For this review, use the dimensioned drawing (mm, ordinates from the lowest corner) and the shaded views. Round coordinates to 2 decimals unless told otherwise and drop trailing zeros. Write each loop counter-clockwise with the first axis right and the second up, starting at its lowest first coordinate (ties: lowest second). Pieces come first, ordered by that corner, then holes.
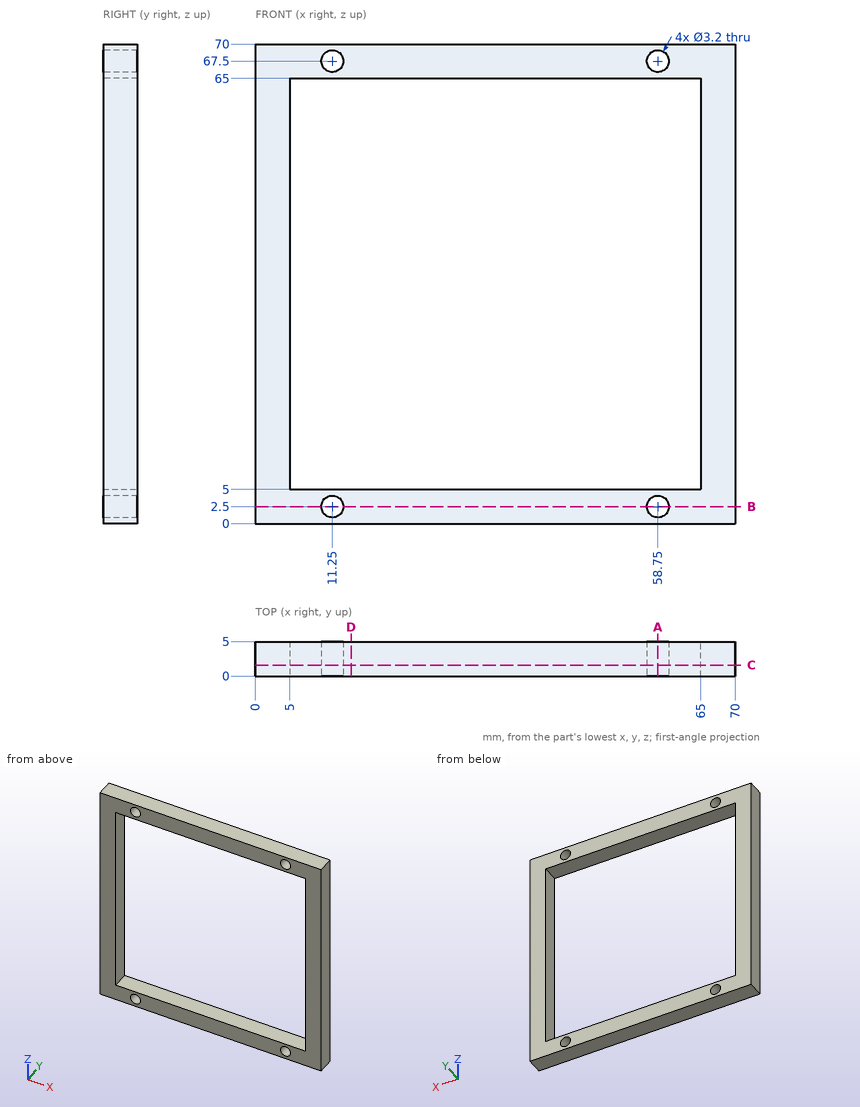
(1) We need section C-C, the plane y = 1.6. Give the boundary of the cut face in (x, z), and give its area (3 significant figures).
Geometry check:
outline: (0, 0) - (70, 0) - (70, 70) - (0, 70) - close; hole (5, 5) - (65, 5) - (65, 65) - (5, 65) - close; hole circle Ø3.2 at (11.25, 2.5); hole circle Ø3.2 at (11.25, 67.5); hole circle Ø3.2 at (58.75, 2.5); hole circle Ø3.2 at (58.75, 67.5)
area: 1,270 mm2
(2) For line 1 along Z through (x, y) = (58.75, 3.95); line 2 along X through (y, z) = (3.75, 51), list the stretches that pass through material, from the lowest coordinate up.
Geometry check:
line 1: z = 0 to 0.9, 4.1 to 5, 65 to 65.9, 69.1 to 70
line 2: x = 0 to 5, 65 to 70
(3) For pin 1 Ø1.9 at (x, z) = (58.75, 67.5) entering from -Y; pin 2 Ø1 at (y, z) = (3, 57) entering from -X, all flat-tipped, find the tip position at first contact; note any pin that passes through.
Geometry check:
pin 1: passes through
pin 2: stops at x = 0
(4) We need section D-D, the plane x = 14. Give the boundary of the cut face in (y, z), and give its area (3 significant figures).
Geometry check:
outline: (0, 0) - (5, 0) - (5, 5) - (0, 5) - close; (0, 65) - (5, 65) - (5, 70) - (0, 70) - close
area: 50.0 mm2
(5) We need section B-B, the plane z = 2.5. Give the boundary of the cut face in (x, y), and give its area (3 significant figures).
Geometry check:
outline: (0, 0) - (9.65, 0) - (9.65, 5) - (0, 5) - close; (12.85, 0) - (57.15, 0) - (57.15, 5) - (12.85, 5) - close; (60.35, 0) - (70, 0) - (70, 5) - (60.35, 5) - close
area: 318 mm2
(6) We need section A-A, the plane x = 58.75. Give the boundary of the cut face in (y, z), and give its area (3 significant figures).
Geometry check:
outline: (0, 0) - (5, 0) - (5, 0.9) - (0, 0.9) - close; (0, 4.1) - (5, 4.1) - (5, 5) - (0, 5) - close; (0, 65) - (5, 65) - (5, 65.9) - (0, 65.9) - close; (0, 69.1) - (5, 69.1) - (5, 70) - (0, 70) - close
area: 18.0 mm2
